Read the model definition and answer for the solid it produces. Units are mm, in the model's axes. Face numbers are marked on the shaded views. Give positions to 0.01 mm unless a question says otherwise; leave off trailing zeros. Write each loop counter-clockwise with the first axis right and the second up, starting at its lowest first coordinate (ties: lowest second). Pieces come first, ordered by that corner, then holes. Notation, with made-up numbers: (-27.5, 42.25) -> (2.5, 42.25) arc R20 ccw to (2.5, 57.25) -> close; hole circle Ø3 at (46.5, 32.25). An arc over 180 degrees is marked (long way). Put each result on its own line as item: value. Start each with the question number.
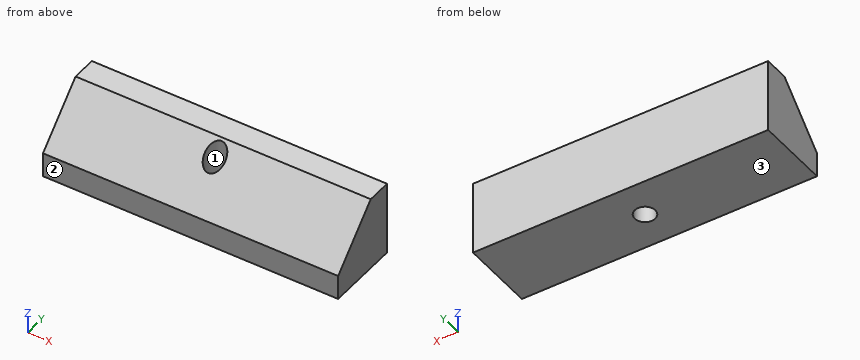
Solid Edge part; units mm, degrees
sketch "Sketch1" plane through (0, 0, 0) normal (0, 0, 1) x (1, 0, 0)
  line L0 (0, 0) -> (0, 9.525)
  line L1 (0, 9.525) -> (38.1, 9.525)
  line L2 (38.1, 9.525) -> (38.1, 0)
  line L3 (38.1, 0) -> (0, 0)
  dimension "D1" = 38.1
extrude "Protrusion1" add sketch "Sketch1" along normal blind 9.525
hole "Hole_1" at (19.05, 4.7625, 0) direction (0, 0, 1) diameter 2.6467 end up to next
chamfer "Chamfer_1" distance 6.35 angle 45 1 edges at (19.05, 0, 9.525)
1) A cutting plane is placed at C-C on x = 19.05. Give the vertices of the cut face in (y, z) (3 decimals).
2) A cutting plane is placed at A-A on y = 4.5. Give the vertices of the cut face in (x, z) (3 decimals).
3) Each of these flat-tipped pins is pushed along its axis until it touches: pin 1 Ø1 at (x, z) = (10, 2) entering from -Y; pin 2 Ø3 at (x, y) = (23, 1.5) entering from +Z (3 decimals); pin 3 Ø2 at (x, y) = (23, 2.5) entering from +Z (3 decimals). Where does it stop, or does it pass through?
4) Straight lines are drawn through the part: line 1 (Y direction, x = 19.05, z = 2.25) (3 decimals); line 2 (Y direction, x = 19.05, z = 3.5) (3 decimals); line 3 (X direction, y = 5, z = 5.5). For each, find the intervals that lie inside material, in ascending order. Write a range as [from, to].
5) For a pull along Y with two mould halves and no side action, classify the marked faces 1, 2 and 3 as pulls with the +Y half, pulls with the -Y half, needs draft (parallel to the pull), parting line crosses it, or undercut.
Results found:
1. outline: (0, 0) -> (3.439, 0) -> (3.439, 6.614) -> (0, 3.175) -> close; (6.086, 0) -> (9.525, 0) -> (9.525, 9.525) -> (6.35, 9.525) -> (6.086, 9.261) -> close
2. outline: (0, 0) -> (17.753, 0) -> (17.753, 7.675) -> (0, 7.675) -> close; (20.347, 0) -> (38.1, 0) -> (38.1, 7.675) -> (20.347, 7.675) -> close
3. pin 1: stops at y = 0
3. pin 2: stops at z = 6.175
3. pin 3: stops at z = 6.675
4. line 1: y = [0, 3.439], [6.086, 9.525]
4. line 2: y = [0.325, 3.439], [6.086, 9.525]
4. line 3: x = [0, 17.75], [20.35, 38.1]
5. face 1: undercut
5. face 2: pulls with the -Y half
5. face 3: needs draft
